Could you check a few things on this model? Use its own coordinates, in mm. A direction names the side the tool comes from. Round coordinates to 2 decimals unless told otherwise and drop trailing zeros. Loops run counter-clockwise (first coordinate to the right, second up) from the corner with the lowest first, then second, coordinate; pieces in that order, holes last.
from build123d import *

# Parameters (mm, degrees)
CROQUIS1_W              = 140
CROQUIS1_H              = 140
CROQUIS1_R              = 1.5
SALIENTE_EXTRUIR1_DEPTH = 5


with BuildPart() as part:
    # Croquis1 → Saliente-Extruir1 (new body)
    with BuildSketch(Plane(origin=(0, 0, 0), x_dir=(1, 0, 0), z_dir=(0, 1, 0))):
        Rectangle(CROQUIS1_W, CROQUIS1_H)
        with Locations(Location((-61, 61, 0), (0, 0, 270))):
            Circle(CROQUIS1_R, mode=Mode.SUBTRACT)
        with Locations(Location((66, 61, 0), (0, 0, 270))):
            Circle(CROQUIS1_R, mode=Mode.SUBTRACT)
        with Locations(Location((66, -61, 0), (0, 0, 270))):
            Circle(CROQUIS1_R, mode=Mode.SUBTRACT)
        with Locations(Location((-61, -61, 0), (0, 0, 270))):
            Circle(CROQUIS1_R, mode=Mode.SUBTRACT)
        with Locations(Location((66, 30.5, 0), (0, 0, 270))):
            Circle(CROQUIS1_R, mode=Mode.SUBTRACT)
        with Locations(Location((66, -30.5, 0), (0, 0, 270))):
            Circle(CROQUIS1_R, mode=Mode.SUBTRACT)
        with Locations(Location((-30.5, -66, 0), (0, 0, 270))):
            Circle(CROQUIS1_R, mode=Mode.SUBTRACT)
        with Locations(Location((30.5, -66, 0), (0, 0, 270))):
            Circle(CROQUIS1_R, mode=Mode.SUBTRACT)
        with Locations(Location((-30.5, 66, 0), (0, 0, 90))):
            Circle(CROQUIS1_R, mode=Mode.SUBTRACT)
        with Locations(Location((30.5, 66, 0), (0, 0, 90))):
            Circle(CROQUIS1_R, mode=Mode.SUBTRACT)
        with Locations(Location((-66, 30.5, 0), (0, 0, 90))):
            Circle(CROQUIS1_R, mode=Mode.SUBTRACT)
        with Locations(Location((-66, -30.5, 0), (0, 0, 90))):
            Circle(CROQUIS1_R, mode=Mode.SUBTRACT)
        Polygon((-55, -62.5), (-62.5, -55), (-62.5, 55), (-55, 62.5), (55, 62.5), (62.5, 55), (62.5, -55), (55, -62.5), align=None, mode=Mode.SUBTRACT)
    extrude(amount=SALIENTE_EXTRUIR1_DEPTH)


solid = part.part
Item 1: If we section it at A-A, the plane x = -17: Please give me the cut outline in (y, z), then the cut area to 3 significant figures.
Results list:
outline: (0, -70) - (5, -70) - (5, -62.5) - (0, -62.5) - close; (0, 62.5) - (5, 62.5) - (5, 70) - (0, 70) - close
area: 75.0 mm2
Item 2: If we section it at C-C, the plane z = 23: Please give me the cut outline in (x, y), then the cut area to 3 significant figures.
Results list:
outline: (-70, 0) - (-62.5, 0) - (-62.5, 5) - (-70, 5) - close; (62.5, 0) - (70, 0) - (70, 5) - (62.5, 5) - close
area: 75.0 mm2
Item 3: We'd pull the mould along Z, two halves only. Please class faces 1 (the flat face through (-1, 2, -62.5)), 2 (the flat face through (-1, 2, -70)), 3 (the flat face through (-63, 5, -11)): released by +Z, released by -Z, zero draft, split by the parting line, or undercut.
Results list:
face 1: undercut
face 2: released by -Z
face 3: zero draft
Item 4: If we section it at B-B, the plane y = 4.05: Count the separate pieces of the cut face and the enclosed holes in it, then the cut area to 3 significant figures.
Results list:
separate pieces: 1
enclosed holes: 13
area: 4,000 mm2
Item 5: If I drill on line 1 along X through (y, z) = (2.6, 66); line 2 along Z through (x, y) = (66, 2.75); line 3 along Z through (x, y) = (52, 1.2), over which ranges is the centre line in solid material (lowest first)?
Results list:
line 1: x = -70 to -32, -29 to 29, 32 to 70
line 2: z = -70 to -62.5, -59.5 to -32, -29 to 29, 32 to 59.5, 62.5 to 70
line 3: z = -70 to -62.5, 62.5 to 70
Item 6: For faces 4 (the flat face through (-63, 0, -11)), 5 (the flat face through (-58.8, 2.5, -58.7)), which set-ups out of +Z, -Z, +X, -X, +Y, -Y let a thin tool reach every point of the face, with its end or its side?
Results list:
face 4: +Z, -Z, +X, -X, -Y
face 5: +Y, -Y
